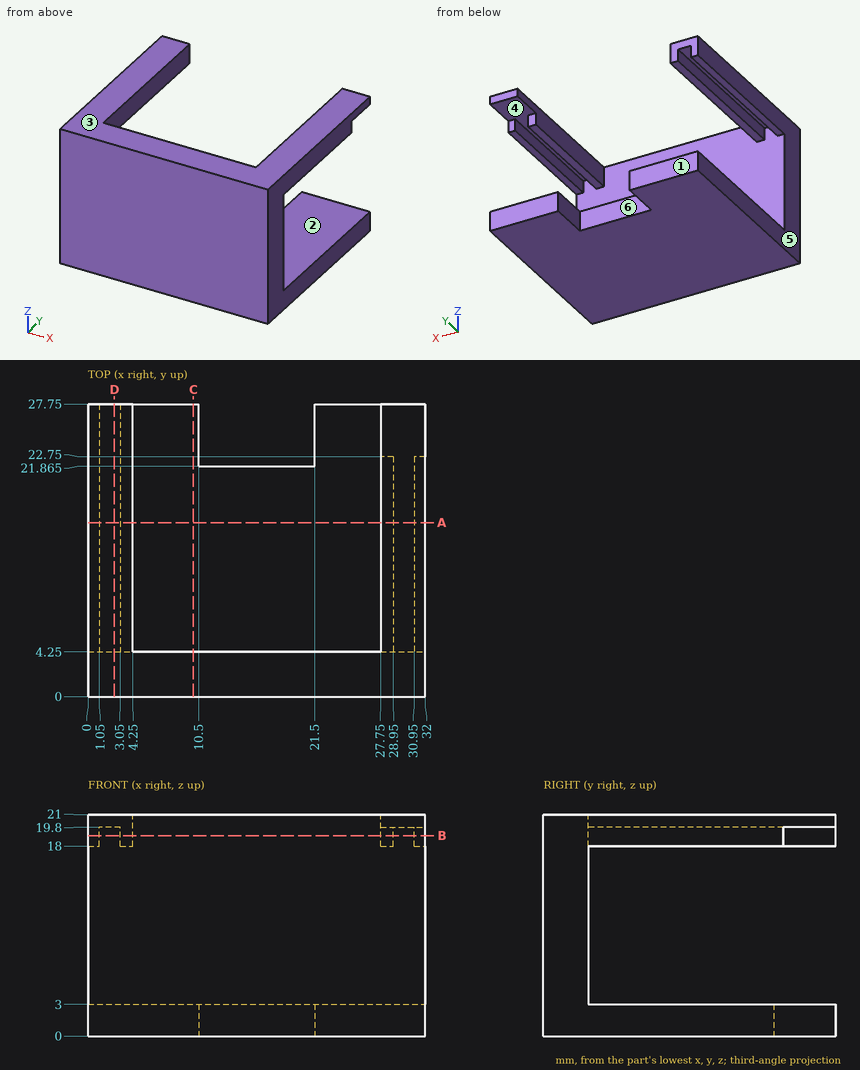
Geometry: see drawing. Coordinates: mm, zero at the bounding-box minimum. A direction names the side the tool comes from. Give positions to 0.01 mm unless a question says otherwise; leave off trailing zeros. Write each loop counter-clockwise with the first axis right and the second up, starting at its lowest first coordinate (ties: lowest second). Pieces come first, ordered by that corner, then holes. Notation, with made-up numbers: M 32,55.25 L 51,55.25 A27 ccw 51,89.25 Z; hole C 41.25,17 d6. An arc over 180 degrees is marked long. Answer in a Markdown table with one row per item. Add a question column.
(1) Reachability of the marked faces 1 and 2 from +Z, -Z, +X, -X, +Y, -Y: full face, straight path, thin tool, end or side. Return the list, or none.
(2) Section C-C on x = 10. Return loops of the section in (y, z).
(3) Section D-D on x = 2.5. Return loops of the section in (y, z).
(4) First-contact query: pin 1 (3 mm diameter, centred on x = 12.5, y = 19.5, fed in from +Z); pin 2 (1.2 mm diameter, centred on x = 31.5, z = 18.5, fed in from +Y); pin 3 (8 mm diameter, centred on x = 16, z = 5.5, fed in from +Y) (1 decimal). Flat tips, straight axial feed; report the tip coordinate or a pass-through.
(5) Ray query, line 1 (Z direction, x = 6.5, y = 7); line 2 (Y direction, x = 4, z = 12.75). Return the intervals inside material, ascending.
(6) Section A-A on y = 16.5. Return loops of the section in (x, z), and give its area (3 significant figures).
(7) Mould query, pull axis X, two halves, no side actions, for the marked faces 3, 4, 5 and 6. Classes: +X half, -X half, draft (parallel to the pull), parting line (faces both ways), or undercut.
(8) Section B-B on z = 19. Return loops of the section in (x, y).
Result set:
| question | item | result |
|---|---|---|
| 1 | face 1 | +Z, -Z, +X, -X, +Y |
| 1 | face 2 | +X, -X, +Y |
| 2 | outline | M 0,0 L 27.75,0 L 27.75,3 L 4.25,3 L 4.25,21 L 0,21 Z |
| 3 | outline | M 0,0 L 27.75,0 L 27.75,3 L 4.25,3 L 4.25,19.8 L 27.75,19.8 L 27.75,21 L 0,21 Z |
| 4 | pin 1 | stops at z = 3 |
| 4 | pin 2 | stops at y = 22.75 |
| 4 | pin 3 | stops at y = 21.9 |
| 5 | line 1 | z = 0 to 3 |
| 5 | line 2 | y = 0 to 4.25 |
| 6 | outline | M 0,0 L 32,0 L 32,3 L 0,3 Z; M 0,18 L 1.05,18 L 1.05,19.8 L 3.05,19.8 L 3.05,18 L 4.25,18 L 4.25,21 L 0,21 Z; M 27.75,18 L 28.95,18 L 28.95,19.8 L 30.95,19.8 L 30.95,18 L 32,18 L 32,21 L 27.75,21 Z |
| 6 | area | 114 mm^2 |
| 7 | face 3 | draft |
| 7 | face 4 | undercut |
| 7 | face 5 | -X half |
| 7 | face 6 | undercut |
| 8 | outline | M 0,0 L 32,0 L 32,22.75 L 30.95,22.75 L 30.95,4.25 L 28.95,4.25 L 28.95,22.75 L 27.75,22.75 L 27.75,4.25 L 4.25,4.25 L 4.25,27.75 L 3.05,27.75 L 3.05,4.25 L 1.05,4.25 L 1.05,27.75 L 0,27.75 Z |
